Source: CAD feature listing. Evaluate the final solid. Frame: model axes, mm. A direction names the side the tool comes from. Give positions to 0.01 mm unless a question says otherwise; leave off trailing zeros. Loops run counter-clockwise (first coordinate to the right, second up) from the corner with the lowest first, then second, coordinate; pieces in that order, holes last. Notation, with made-up numbers: (62.5, 79) -> (79.5, 79) arc R17 ccw to (79.5, 83) -> close; hole circle Ø2 at (3.25, 14.5). An arc over 180 degrees is marked (long way). Put each result on its own line as item: value.
```python
from build123d import *

# Parameters (mm, degrees)
ESQUISSE1_R        = 29.281018542
BOSS_EXTRU_1_DEPTH = 125
ESQUISSE2_R        = 10
BOSS_EXTRU_2_DEPTH = 25


with BuildPart() as part:
    # Esquisse1 → Boss.-Extru.1 (new body)
    with BuildSketch(Plane.XY):
        with BuildLine():
            Line((25, 37.416573868), (-25, 37.416573868))
            ThreePointArc((-25, 37.416573868), (-45, 0), (-25, -37.416573868))
            Line((-25, -37.416573868), (25, -37.416573868))
            ThreePointArc((25, -37.416573868), (39.686269666, -21.213203436), (45, 0))
            ThreePointArc((45, 0), (39.686269666, 21.213203436), (25, 37.416573868))
        make_face()
        Circle(ESQUISSE1_R, mode=Mode.SUBTRACT)
    extrude(amount=BOSS_EXTRU_1_DEPTH)

    # Esquisse2 → Boss.-Extru.2 (add)
    with BuildSketch(Plane(origin=(0, 37.416573868, 0), x_dir=(1, 0, 0), z_dir=(0, 1, 0))):
        with Locations(Location((0, -62.5, 0), (0, 0, 270))):
            Circle(ESQUISSE2_R)
    boss_extru_2 = extrude(amount=BOSS_EXTRU_2_DEPTH)

    # Symétrie1: Boss.-Extru.2 across plane
    add(boss_extru_2.mirror(Plane.ZX))


solid = part.part
```
(1) Section A-A on x = 0. Return loops of the section in (y, z).
Calculated:
outline: (-62.42, 52.5) -> (-37.42, 52.5) -> (-37.42, 0) -> (-29.28, 0) -> (-29.28, 125) -> (-37.42, 125) -> (-37.42, 72.5) -> (-62.42, 72.5) -> close; (29.28, 0) -> (37.42, 0) -> (37.42, 52.5) -> (62.42, 52.5) -> (62.42, 72.5) -> (37.42, 72.5) -> (37.42, 125) -> (29.28, 125) -> close
(2) Reachability of faces 5 (the flat face through (0, 62.417, 62)), 6 (the cylindrical face through (0.44, -49.74, 52.51)) from +Z, -Z, +X, -X, +Y, -Y: full face, straight path, thin tool, end or side. Return the list, or none.
Calculated:
face 5: +Z, -Z, +X, -X, +Y
face 6: -Y
(3) Section D-D on x = 23. Return loops of the section in (y, z), then the cut area to 3 significant figures.
Calculated:
outline: (-37.42, 0) -> (-18.12, 0) -> (-18.12, 125) -> (-37.42, 125) -> close; (18.12, 0) -> (37.42, 0) -> (37.42, 125) -> (18.12, 125) -> close
area: 4,820 mm²
(4) Section C-C on y = -6.5. Return loops of the section in (x, z), then the cut area to 3 significant figures.
Calculated:
outline: (-44.53, 0) -> (-28.55, 0) -> (-28.55, 125) -> (-44.53, 125) -> close; (28.55, 0) -> (44.53, 0) -> (44.53, 125) -> (28.55, 125) -> close
area: 3,990 mm²
(5) Draft query along X for faces 1 (the cylindrical face through (0.44, 49.74, 52.51)), 2 (the flat face through (11, 37.417, 62)), 3 (the cylindrical face through (27.929, 8.795, 61.625)), 4 (the cylindrical face through (-44.996, 0.618, 61.625)). Return one class per face: released by +X, released by -X, zero draft, split by the parting line, or undercut.
Calculated:
face 1: split by the parting line
face 2: zero draft
face 3: undercut
face 4: released by -X
(6) Section B-B on z = 62.5. Return loops of the section in (x, y), then the cut area to 3 significant figures.
Calculated:
outline: (-25, -37.42) -> (-10, -37.42) -> (-10, -62.42) -> (10, -62.42) -> (10, -37.42) -> (25, -37.42) arc R45 ccw to (25, 37.42) -> (10, 37.42) -> (10, 62.42) -> (-10, 62.42) -> (-10, 37.42) -> (-25, 37.42) arc R45 ccw to start; hole circle Ø58.56 at (0, 0)
area: 4,150 mm²
(7) First-contact query: P1, Ø8, axis at x = -13, z = 40, coming from the -Y side; P2, Ø2, axis at y = 16, z = 47, coming from the +X side; P3, Ø1, axis at x = 14, z = 34.5, coming from the +Y side. Flat tips, straight axial feed; report the tip coordinate or a pass-through.
Calculated:
P1: stops at y = -37.42
P2: stops at x = 42.43
P3: stops at y = 37.42
(8) Line query: probe 1 along Y at (x, z) = (0, 86.5); probe 2 along Y at (x, z) = (0, 68); probe 3 along X at (y, z) = (-14, 67). Output: solid intervals per line, ascending. Write a range as from..to.
Calculated:
probe 1: y = -37.42..-29.28, 29.28..37.42
probe 2: y = -62.42..-29.28, 29.28..62.42
probe 3: x = -42.77..-25.72, 25.72..42.77
